Check sheet for the drawn part. Datum: minimum x, y, z corner. Units: mm. A direction names the side the tool comes from. Round coordinates to 2 decimals unless told otherwise and drop trailing zeros. Write each loop counter-clockwise with the first axis right and the second up, starting at its lowest first coordinate (ties: lowest second). Pieces come first, ordered by that corner, then holes. Notation, with made-up numbers: (-6.5, -28) - (37.5, -28) arc R21 ccw to (37.5, 3) - close; hole circle Ø11 at (-5, 81). An arc over 180 degrees is marked (long way). Write each question's results on one line, items separated by ' | '.
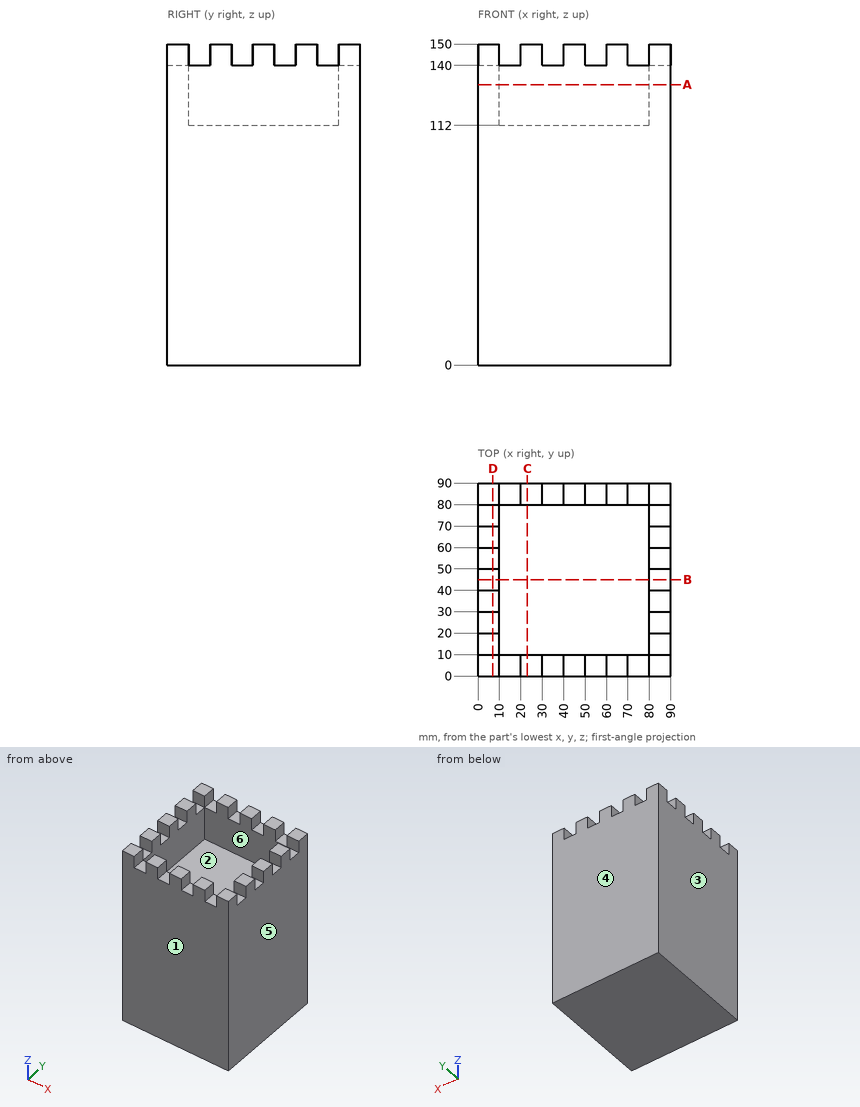
(1) Thickness scan on L1, parallel to X at y = 13.5, z = 128.5; L2, parallel to Z at x = 29.5, y = 20. Record the ranges inside material, lowest first.
Answer:
L1: 0 to 10, 80 to 90 | L2: 0 to 112
(2) Section check D-D (x = 7). Record the cut outline in (y, z), plus the area to 3 significant figures.
Answer:
outline: (0, 0) - (90, 0) - (90, 150) - (80, 150) - (80, 140) - (70, 140) - (70, 150) - (60, 150) - (60, 140) - (50, 140) - (50, 150) - (40, 150) - (40, 140) - (30, 140) - (30, 150) - (20, 150) - (20, 140) - (10, 140) - (10, 150) - (0, 150) - close | area: 13,100 mm2
(3) Go/stop test with flat-tipped pins: pin 1 Ø8 at (x, y) = (17.5, 39.5) entering from +Z; pin 2 Ø11 at (y, z) = (4, 144.5) entering from -X; pin 3 Ø5 at (x, y) = (55.5, 6) entering from +Z. Record where each tip stops, or that it passes through.
Answer:
pin 1: z = 112 | pin 2: x = 0 | pin 3: z = 140
(4) Set-up check for the marked faces 5 and 6: record each of +Z, -Z, +X, -X, +Y, -Y from which the full face is reachable in a straight line by a thin tool's end or side.
Answer:
face 5: +Z, -Z, +X, +Y, -Y | face 6: +Z
(5) Mould release check, pull along Y, two halves, no side actions. Record for the marked faces 1, 2, 3 and 4: released by +Y, released by -Y, zero draft, split by the parting line, or undercut.
Answer:
face 1: released by -Y | face 2: undercut | face 3: zero draft | face 4: released by +Y
(6) Section check B-B (y = 45). Record the cut outline in (x, z), plus the area to 3 significant figures.
Answer:
outline: (0, 0) - (90, 0) - (90, 150) - (80, 150) - (80, 112) - (10, 112) - (10, 150) - (0, 150) - close | area: 10,800 mm2
(7) Section check A-A (z = 131). Record the cut outline in (x, y).
Answer:
outline: (0, 0) - (90, 0) - (90, 90) - (0, 90) - close; hole (10, 10) - (80, 10) - (80, 80) - (10, 80) - close
